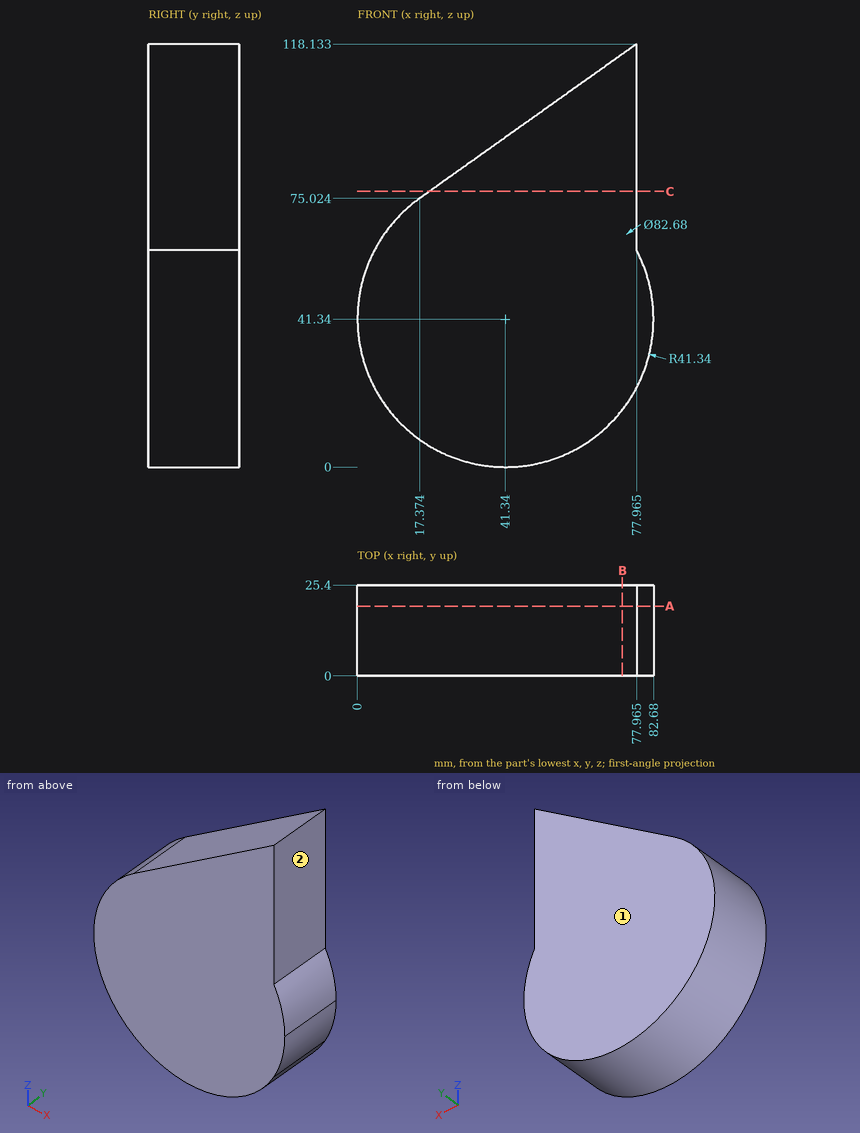
Source: three-view drawing plus pictorial views. Frame: mm from the lowest corner of the part. A direction names the side the tool comes from. Give positions to 0.01 mm unless a question says otherwise; leave off trailing zeros. Write each loop counter-clockwise with the first axis right and the second up, starting at its lowest first coordinate (ties: lowest second). Pieces come first, ordered by that corner, then holes. Notation, with made-up numbers: (23, 14.25) -> (64, 14.25) arc R15 cw to (64, 41.25) -> close; hole circle Ø9 at (87, 69.25). An arc over 180 degrees is marked (long way). Answer in a Markdown table with one row per item.
(1) Section query B-B on x = 74. Return loops of the section in (y, z).
Answers below:
| item | result |
|---|---|
| outline | (0, 16) -> (25.4, 16) -> (25.4, 115.31) -> (0, 115.31) -> close |
(2) Set-up query: the marked faces 1 and 2. Return all of +Z, -Z, +X, -X, +Y, -Y with unobstructed straight access to the full face (end or side cutting, diameter ignored); none if empty.
Answers below:
| item | result |
|---|---|
| face 1 | +Z, -Z, +X, -X, +Y |
| face 2 | +Z, +X, +Y, -Y |
(3) Ray query, line 1 along X through (y, z) = (4, 40.5); line 2 along X through (y, z) = (17.5, 98.5) (1 decimal); line 3 along Z through (x, y) = (66, 1.75). Return the intervals inside material, ascending. Write a range as [from, to].
Answers below:
| item | result |
|---|---|
| line 1 | [0.01, 82.67] |
| line 2 | [50.4, 78] |
| line 3 | [8.16, 109.62] |
(4) Section query C-C on z = 77. Return loops of the section in (x, y) (1 decimal), then the cut area to 3 significant figures.
Answers below:
| item | result |
|---|---|
| outline | (20.2, 0) -> (78, 0) -> (78, 25.4) -> (20.2, 25.4) -> close |
| area | 1,470 mm^2 |
(5) Section query A-A on y = 19.5. Return loops of the section in (x, z) (1 decimal).
Answers below:
| item | result |
|---|---|
| outline | (17.4, 75) arc R41.3 ccw (long way) to (77.9, 22.1) arc R41.3 ccw to (82.7, 41.3) arc R41.3 ccw to (78, 60.5) -> (78, 118.1) -> close |
(6) Pin query (flat end, axial travel): pin 1 (3 mm diameter, centred on x = 40.5, z = 92.5, fed in from -Y); pin 2 (12.5 mm diameter, centred on y = 17, z = 92, fed in from +X) (1 decimal); pin 3 (10 mm diameter, centred on y = 21, z = 81.5, fed in from -X); pin 4 (1 mm diameter, centred on y = 16.5, z = 59.5, fed in from +X). Return the tip coordinate at first contact, or that it passes through.
Answers below:
| item | result |
|---|---|
| pin 1 | y = 0 |
| pin 2 | x = 78 |
| pin 3 | x = 19.45 |
| pin 4 | x = 78.72 |
